The model under review builds one solid part; all positions refer to its coordinate system, in mm. Face numbers are marked on the shaded views. Round coordinates to 2 decimals unless told otherwise and drop trailing zeros. Loops run counter-clockwise (first coordinate to the right, second up) from the corner with the lowest first, then second, coordinate; pieces in that order, holes last. Notation, with made-up numbers: M 59,53.25 L 74,53.25 A23 ccw 74,79.25 Z; hole C 6.25,-0.5 d4. An arc over 180 degrees is marked long. Answer as a JSON object with one key per item and string values. Group by question number.
Item 1: Insertion check: P1, Ø0.8, axis at y = -11.5, z = 49.5, coming from the +X side; P2, Ø0.6, axis at y = 11, z = 49.5, coming from the -X side; P3, Ø8, axis at x = 8, y = -2, coming from the -Z side. Each pin has a flat end and moves straight along its axis. Give the tip position at first contact, or say it passes through.
Item 2: Consider section B-B (x = -0.5). Give the boundary of the cut face in (y, z), and give its area (3 significant figures).
Item 3: Consider section C-C (z = 52.1). Give the boundary of the cut face in (x, y).
Item 4: Consider section A-A (y = 8.5). Give the boundary of the cut face in (x, z).
Item 5: The part is to be moulded in two halves that separate along Y. For the marked faces 1, 2 and 3, say which applies: +Y half, -Y half, draft (parallel to the pull), parting line (faces both ways), or undercut.
Item 6: To check wall thickness, follow line 1 (X direction, y = -9.75, z = 49.8); line 2 (Y direction, x = 12, z = 49.45); line 3 (Z direction, x = 10, y = 9). State the ranges of each line that lie inside material, in increasing order.
```python
from build123d import *

# Parameters (mm, degrees)
SKETCH046_W     = 31.5
SKETCH046_H     = 20
PAD026_DEPTH    = 2
THICKNESS008_T  = 1.5
SKETCH050_W     = 33
SKETCH050_H     = 21.5
POCKET016_DEPTH = 5
POCKET017_DEPTH = 1


with BuildPart() as part:
    # Sketch046 → Pad026 (new body)
    with BuildSketch(Plane.XY):
        Rectangle(SKETCH046_W, SKETCH046_H)
    extrude(amount=PAD026_DEPTH)

    # Thickness008
    thickness008_openings = [part.faces().sort_by_distance(p)[0] for p in [
        (0, 0, 0),
    ]]
    offset(amount=THICKNESS008_T, openings=thickness008_openings)

    # Sketch050 (on Face5 of Thickness008) → Pocket016 (cut)
    with BuildSketch(Plane(origin=(0, 0, 2), x_dir=(1, 0, 0), z_dir=(0, 0, -1))):
        Rectangle(SKETCH050_W, SKETCH050_H)
    extrude(amount=POCKET016_DEPTH, mode=Mode.SUBTRACT)

    # Sketch048 → Pocket017 (cut)
    with BuildSketch(Plane.XY):
        Polygon((-28.138837, 2.5), (-2.5, 2.5), (-2.5, 15.913807), (2.5, 15.913807), (2.5, 2.5), (28.138837, 2.5), (28.138837, -2.5), (2.5, -2.5), (2.5, -15.913807), (-2.5, -15.913807), (-2.5, -2.5), (-28.138837, -2.5), align=None)
    extrude(amount=POCKET017_DEPTH, mode=Mode.SUBTRACT)


with BuildPart() as part_1:
    # Body011 placement: moved
    add(part.part.moved(Location((0, 0, 49))))


solid = part_1.part
```
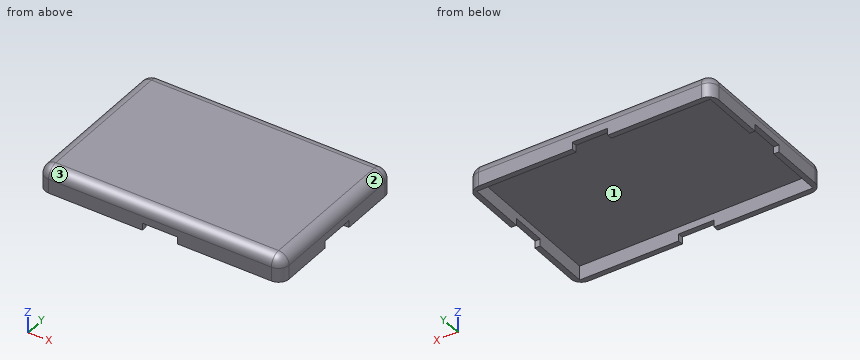
Geometry results:
{
 "1": {"P1": "stops at x = 16.77", "P2": "stops at x = -17.08", "P3": "stops at z = 51"},
 "2": {"outline": "M -11.5,50 L -10.75,50 L -10.75,51 L 10.75,51 L 10.75,50 L 11.5,50 L 11.5,51 A1.5 ccw 10,52.5 L -10,52.5 A1.5 ccw -11.5,51 Z", "area": "35.0 mm^2"},
 "3": {"outline": "M -16.77,-10 A1.02 ccw -15.75,-11.02 L 15.75,-11.02 A1.02 ccw 16.77,-10 L 16.77,10 A1.02 ccw 15.75,11.02 L -15.75,11.02 A1.02 ccw -16.77,10 Z"},
 "4": {"outline": "M -17.25,49 L -16.5,49 L -16.5,51 L 16.5,51 L 16.5,49 L 17.25,49 L 17.25,51 A1.5 ccw 15.75,52.5 L -15.75,52.5 A1.5 ccw -17.25,51 Z"},
 "5": {"face 1": "undercut", "face 2": "draft", "face 3": "-Y half"},
 "6": {"line 1": "x = -17.25 to -16.5, 16.5 to 17.25", "line 2": "y = -11.5 to -10.75, 10.75 to 11.5", "line 3": "z = 51 to 52.5"}
}
